Drawing for the job (mm, zero at the part's lowest x, y, z). Give positions to 0.01 mm unless a question says otherwise; leave off trailing zeros. Order: outer loops, then holes, each group sorted by start corner. A loop starts at its lowest first (then second) coordinate and runs counter-clockwise, first axis right, second up. Notation, with made-up numbers: (-21, 10.5) - (34, 10.5) arc R28 cw to (34, 40.5) - close; hole circle Ø5 at (28, 18). An arc over 180 degrees is marked (long way). One line per item, written item: value.
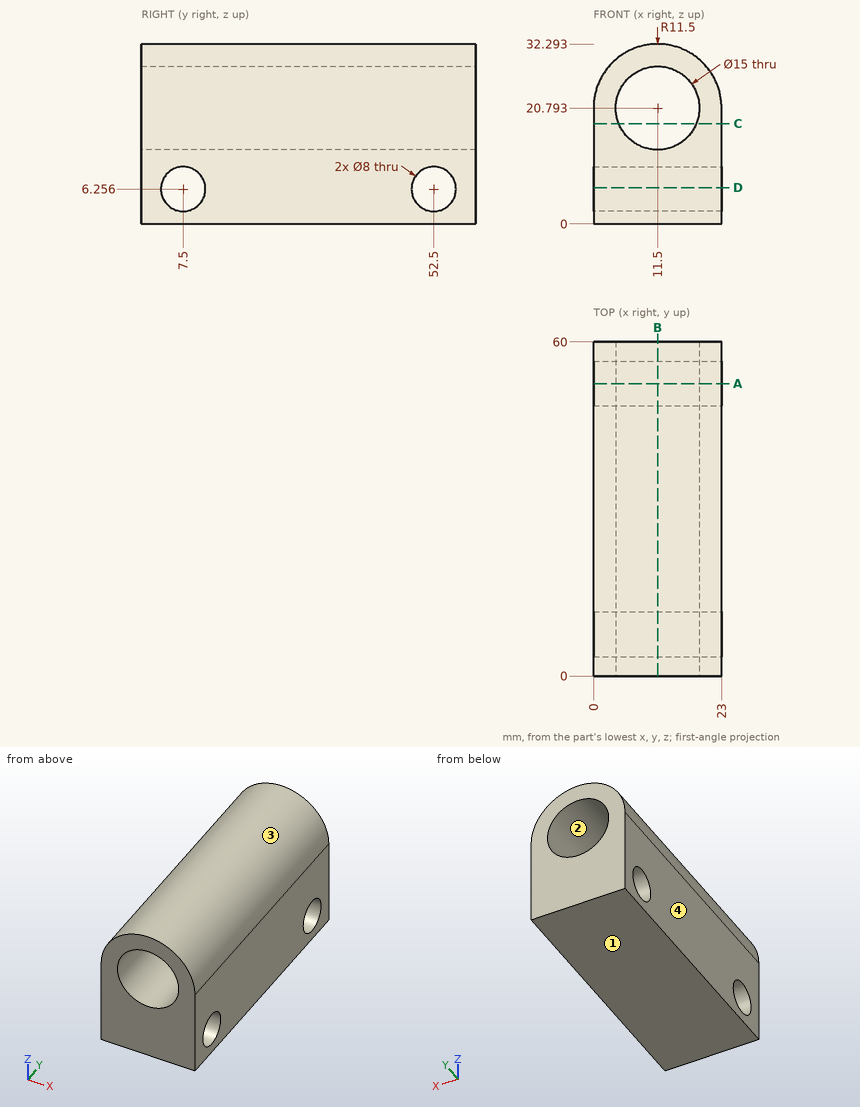
1) Mould opens along X. For the marked faces 1, 2, 3 and 4 say: released by +X, released by -X, zero draft, split by the parting line, or undercut.
Outcome:
face 1: zero draft
face 2: undercut
face 3: split by the parting line
face 4: released by -X
2) Cut at C-C, the plane z = 18. Give the cut face in (x, y).
Outcome:
outline: (0, 0) - (4.54, 0) - (4.54, 60) - (0, 60) - close; (18.46, 0) - (23, 0) - (23, 60) - (18.46, 60) - close
3) Pin check, flat tips, straight feed: pin 1 (5 mm diameter, centred on y = 52.5, z = 6.26, fed in from +X); pin 2 (10.5 mm diameter, centred on y = 7.5, z = 6.26, fed in from -X). Stop position of each tip, or through.
Outcome:
pin 1: passes through
pin 2: stops at x = 0
4) Cut at B-B, the plane x = 11.5. Give the cut face in (y, z).
Outcome:
outline: (0, 0) - (60, 0) - (60, 13.29) - (0, 13.29) - close; (0, 28.29) - (60, 28.29) - (60, 32.29) - (0, 32.29) - close; hole circle Ø8 at (7.5, 6.26); hole circle Ø8 at (52.5, 6.26)
5) Cut at A-A, the plane y = 52.5. Give the cut face in (x, z).
Outcome:
outline: (0, 0) - (23, 0) - (23, 2.26) - (0, 2.26) - close; (0, 10.26) - (23, 10.26) - (23, 20.79) arc R11.5 ccw to (0, 20.79) - close; hole circle Ø15 at (11.5, 20.79)
6) Drill centre lines: line 1 along Z through (x, y) = (11.25, 40.5); line 2 along Z through (x, y) = (5.5, 53) (1 decimal); line 3 along Z through (x, y) = (5.5, 50.5) (1 decimal). Where is each one in solid material? Low to high. Write a range as from..to.
Outcome:
line 1: z = 0..13.3, 28.29..32.29
line 2: z = 0..2.3, 10.2..16.3, 25.3..30.6
line 3: z = 0..2.8, 9.7..16.3, 25.3..30.6
7) Cut at D-D, the plane z = 6.5. Give the cut face in (x, y), then the cut area to 3 significant figures.
Outcome:
outline: (0, 0) - (23, 0) - (23, 3.51) - (0, 3.51) - close; (0, 11.49) - (23, 11.49) - (23, 48.51) - (0, 48.51) - close; (0, 56.49) - (23, 56.49) - (23, 60) - (0, 60) - close
area: 1,010 mm^2
